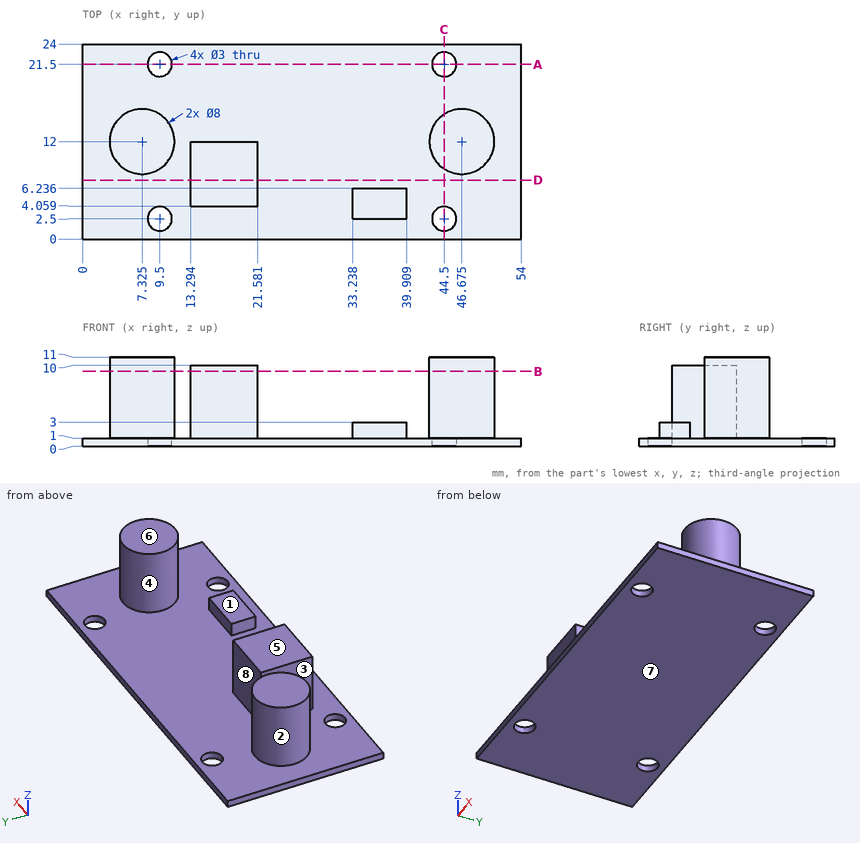
Input: dimensioned drawing with shaded views. Units: mm. Origin: part minimum x, y, z. A direction names the side the tool comes from. Give positions to 0.01 mm unless a question says otherwise; leave off trailing zeros. Loops run counter-clockwise (first coordinate to the right, second up) from the corner with the lowest first, then second, coordinate; pieces in that order, holes last. Notation, with made-up numbers: M -20.5,24.5 L -4.5,24.5 A23 ccw -4.5,42.5 Z; hole C -36,65 d2. An arc over 180 degrees is marked long. Put each result on its own line as item: value.
1) Reachability of the marked faces 4, 5, 6, 7 and 8 from +Z, -Z, +X, -X, +Y, -Y: full face, straight path, thin tool, end or side. Return the list, or none.
Computed values:
face 4: +Z
face 5: +Z, +Y, -Y
face 6: +Z, +X, -X, +Y, -Y
face 7: -Z, +X, -X, +Y, -Y
face 8: +Z, +Y
2) Cut plane A-A, the plane y = 21.5. Return the cut outline in (x, z).
Computed values:
outline: M 0,0 L 8,0 L 8,1 L 0,1 Z; M 11,0 L 43,0 L 43,1 L 11,1 Z; M 46,0 L 54,0 L 54,1 L 46,1 Z
3) Cut plane B-B, the plane z = 9.25. Return the cut outline in (x, y) (1 decimal), plus the area to 3 significant figures.
Computed values:
outline: C 7.3,12 d8; M 13.3,4.1 L 21.6,4.1 L 21.6,12 L 13.3,12 Z; C 46.7,12 d8
area: 166 mm^2
4) Mould query, pull axis X, two halves, no side actions, for the marked faces 1, 2 and 3. Classes: released by +X, released by -X, zero draft, split by the parting line, or undercut.
Computed values:
face 1: zero draft
face 2: undercut
face 3: undercut
5) Cut plane C-C, the plane x = 44.5. Return the cut outline in (y, z).
Computed values:
outline: M 0,0 L 1,0 L 1,1 L 0,1 Z; M 4,0 L 20,0 L 20,1 L 15.36,1 L 15.36,11 L 8.64,11 L 8.64,1 L 4,1 Z; M 23,0 L 24,0 L 24,1 L 23,1 Z
6) Cut plane D-D, the plane y = 7.25. Return the cut outline in (x, z).
Computed values:
outline: M 0,0 L 54,0 L 54,1 L 21.58,1 L 21.58,10 L 13.29,10 L 13.29,1 L 0,1 Z
7) First-contact query: P1, Ø1.6, axis at x = 36.5, z = 2.5, coming from the -Y side; P2, Ø0.6, axis at y = 4, z = 2, coming from the +X side; P3, Ø4, axis at x = 9.5, y = 2.5, coming from the +Z side. Flat tips, straight axial feed; report the tip coordinate or a pass-through.
Computed values:
P1: stops at y = 2.5
P2: stops at x = 39.91
P3: stops at z = 1
8) Material intervals for L1, parallel to Y at x = 9.5, z = 0.75; L2, parallel to X at y = 10, z = 3.25 (1 decimal); L3, parallel to Z at x = 44, y = 18, sorted ascending. Write a range as from..to.
Computed values:
L1: y = 0..1, 4..20, 23..24
L2: x = 3.9..10.8, 13.3..21.6, 43.2..50.1
L3: z = 0..1
